from build123d import *


with BuildPart() as f1:
    # F0 (on Right) → F1 (revolve)
    with BuildSketch(Plane.YZ):
        Polygon((0, 76.2), (0, 114.3), (-12.7, 114.3), (-12.7, 82.55), (-292.1, 82.55), (-292.1, 114.3), (-304.8, 114.3), (-304.8, 76.2), align=None)
    revolve(axis=Axis((0, 69.986956, 0), (0, 1, 0)))

    # F3 (on mid) → F4 (revolve)
    with BuildSketch(Plane(origin=(0, -152.4, 0), x_dir=(-1, 0, 0), z_dir=(0, 1, 0))):
        Polygon((304.799496, 76.2), (304.799496, 114.3), (292.099496, 114.3), (292.099496, 82.55), (-0.000504, 82.55), (-0.000504, 76.2), align=None)
    revolve(axis=Axis((-10.273844, -152.4, 0), (1, 0, 0)))


solid = f1.part
For this review, take the finished solid that the model builds, in its own axes (mm). A direction names the side the tool comes from. Round coordinates to 2 decimals unless told otherwise and drop trailing zeros. Order: outer loops, then holes, each group sorted by start corner. A loop starts at its lowest first (then second) coordinate and runs counter-clockwise, first axis right, second up. Notation, with made-up numbers: M -2,74 L 6,74 A34 cw 6,105 Z; hole C -18.75,-33 d11. An arc over 180 degrees is marked long. Write each question's results on one line, items separated by ' | '. Start each with the question number.
1. Add section B-B (x = -216.5). State the section outline as (y, z) points, then the cut area to 3 significant figures.
2. Add section A-A (y = -54.5). State the section outline as (x, z) points, then the cut area to 3 significant figures.
3. Draft analysis for pull direction X (two halves, no side actions). For faces 1 (the face through (-29.1, -234.94, 1.36)), 2 (the face through (-304.799, -129, -75)), 3 (the face through (-29.1, -69.86, -1.36)), 4 (the face through (-298.36, -40.82, -24.78)), state which applies: pulls with the +X half, pulls with the -X half, needs draft (parallel to the pull), parting line crosses it, or undercut.
4. Clearance check with flat-ended pins moving along their axes: pin 1 Ø8 at (x, y) = (-139.5, -123.5) entering from -Z; pin 2 Ø1 at (y, z) = (-194.5, 59) entering from +X; pin 3 Ø6 at (x, z) = (-137, 68) entering from +Y. State where each tip first meets the part, or that it passes through.
5. To check wall thickness, follow L1, parallel to Z at x = -230.5, y = -152.4; L2, parallel to Y at x = -261, z = -3; L3, parallel to X at y = -243, z = 0. State the ranges of each line that lie inside material, in increasing order. Write a range as [from, to].
6. Tool access review of faces 5 (the face through (-170.186, -123.215, 70.389)), 6 (the face through (-76.18, -152.17, -1.68)), 7 (the face through (0.001, -75, 0)): name each direction out of +Z, -Z, +X, -X, +Y, -Y from which nothing blocks a thin tool from reaching the whole face with its end or side.
7. Add section C-C (y = -132.5). State the section outline as (x, z) points.
8. Add section D-D (y = -192). State the section outline as (x, z) points.
Output values:
1) outline: C -152.4,0 d165.1; hole C -152.4,0 d152.4 | area: 3,170 mm^2
2) outline: M -304.8,-58.99 L -292.1,-58.99 L -292.1,58.99 L -304.8,58.99 Z; C 0,0 d165.1; hole C 0,0 d152.4 | area: 4,670 mm^2
3) face 1: undercut | face 2: pulls with the -X half | face 3: undercut | face 4: needs draft
4) pin 1: z = -78.71 | pin 2: x = 58.24 | pin 3: y = -101.51
5) L1: [-82.55, -76.2], [76.2, 82.55] | L2: [-234.9, -228.54], [-76.26, -69.9] | L3: [-304.8, -292.1], [-82.55, -76.2], [76.2, 82.55]
6) face 5: -X | face 6: none | face 7: +Y, -Y
7) outline: M -304.8,-112.55 L -292.1,-112.55 L -292.1,-80.12 L -19.9,-80.12 A82.55 ccw long -19.9,80.12 L -292.1,80.12 L -292.1,112.55 L -304.8,112.55 L -304.8,73.56 L -37.47,73.56 A82.55 ccw -37.47,-73.56 L -304.8,-73.56 Z; hole M -19.9,-73.56 L 0,-73.56 L 0,-76.2 A76.2 ccw 0,76.2 L 0,73.56 L -19.9,73.56 A76.2 ccw Z
8) outline: M -304.8,-107.22 L -292.1,-107.22 L -292.1,-72.43 L -39.6,-72.43 A82.55 ccw long -39.6,72.43 L -292.1,72.43 L -292.1,107.22 L -304.8,107.22 L -304.8,65.1 L -50.76,65.1 A82.55 ccw -50.76,-65.1 L -304.8,-65.1 Z; hole M -39.6,-65.1 L 0,-65.1 L 0,-72.43 L -23.67,-72.43 A76.2 ccw long -23.67,72.43 L 0,72.43 L 0,65.1 L -39.6,65.1 A76.2 ccw Z
